from build123d import *

# Parameters (mm, degrees)
SKETCH1_R           = 1.5
BOSS_EXTRUDE1_DEPTH = 6


with BuildPart() as part:
    # Sketch1 → Boss-Extrude1 (new body)
    with BuildSketch(Plane(origin=(0, 0, 0), x_dir=(1, 0, 0), z_dir=(0, 1, 0))):
        with BuildLine():
            Line((-12.5, 10), (0, 10))
            Line((0, 10), (0, -10))
            Line((0, -10), (-12.5, -10))
            ThreePointArc((-12.5, -10), (-22.5, 0), (-12.5, 10))
        make_face()
        with Locations(Location((-12.5, 0, 0), (0, 0, 270))):
            Circle(SKETCH1_R, mode=Mode.SUBTRACT)
    boss_extrude1 = extrude(amount=BOSS_EXTRUDE1_DEPTH)

    # Mirror1: Boss-Extrude1 across plane
    add(boss_extrude1.mirror(Plane(origin=(0, 6, -10), x_dir=(0, 0, 1), z_dir=(-1, 0, 0))))


solid = part.part
Build history of the part. All positions in model axes, mm. Round coordinates to 2 decimals unless told otherwise and drop trailing zeros. Write each loop counter-clockwise with the first axis right and the second up, starting at its lowest first coordinate (ties: lowest second). Pieces come first, ordered by that corner, then holes. Notation, with made-up numbers: M -16.75,-7 L 23.25,-7 A22 ccw 23.25,24 Z; hole C 17,-28.5 d9. An arc over 180 degrees is marked long. Use CSV: the item, a comma, the result in double quotes.
1. Saw through at C-C (z = -6). Give the cut face in (x, y), plus the area to 3 significant figures.
Reply:
outline,"M -20.5,0 L 20.5,0 L 20.5,6 L -20.5,6 Z"
area,"246 mm²"
2. Saw through at D-D (z = 6.25). Give the cut face in (x, y).
Reply:
outline,"M -20.31,0 L 20.31,0 L 20.31,6 L -20.31,6 Z"
3. Flat gauge pins, fed straight in: pin 1 (3 mm diameter, centred on y = 1, z = 6.5, fed in from -X); pin 2 (2 mm diameter, centred on y = 3.5, z = -3.5, fed in from -X). Where does each tip first touch, or does it go through?
Reply:
pin 1,"stops at x = -21.16"
pin 2,"stops at x = -22.18"
4. Saw through at B-B (y = 3.2). Give the cut face in (x, z), plus the area to 3 significant figures.
Reply:
outline,"M -12.5,-10 L 12.5,-10 A10 ccw 12.5,10 L -12.5,10 A10 ccw Z; hole C -12.5,0 d3; hole C 12.5,0 d3"
area,"800 mm²"
5. Two-plate mould, pull along X, no slides. Class faces 1 (the face through (12.05, 2.96, 1.43)), 2 (the face through (-12.05, 2.96, 1.43)), 3 (the face through (-22.5, 3, 0.2)), 4 (the face through (0, 3, -10)): +X half, -X half, draft (parallel to the pull), parting line (faces both ways), or undercut.
Reply:
face 1,"undercut"
face 2,"undercut"
face 3,"-X half"
face 4,"draft"
6. Wall check: probe 1 along X at (y, z) = (1.35, 0); probe 2 along Z at (x, y) = (12.5, 4.65); probe 3 along Z at (x, y) = (20, 1.5). Give the ranges that are in metal, low to high. Write a range as from..to.
Reply:
probe 1,"x = -22.5..-14, -11..11, 14..22.5"
probe 2,"z = -10..-1.5, 1.5..10"
probe 3,"z = -6.61..6.61"
7. Saw through at A-A (z = 0). Give the cut face in (x, y), plus the area to 3 significant figures.
Reply:
outline,"M -22.5,0 L -14,0 L -14,6 L -22.5,6 Z; M -11,0 L 11,0 L 11,6 L -11,6 Z; M 14,0 L 22.5,0 L 22.5,6 L 14,6 Z"
area,"234 mm²"
